Part print with two shaded views. Sizes in mm from the minimum x, y, z corner. A direction names the side the tool comes from. Round coordinates to 2 decimals unless told otherwise and drop trailing zeros. Write each loop counter-clockwise with the first axis right and the second up, starting at its lowest first coordinate (ties: lowest second). Pieces come first, ordered by that corner, then holes. Notation, with made-up numbers: (1.5, 15) - (45.5, 15) arc R17 ccw to (45.5, 20) - close; hole circle Ø3 at (-13, 48). An arc over 180 degrees is marked (long way). Answer as a JSON object with one key per item and string values. Group by question number.
Item 1: Flat gauge pins, fed straight in: pin 1 (1.7 mm diameter, centred on x = 13.25, y = 1.85, fed in from +Z); pin 2 (1.4 mm diameter, centred on x = 3.25, y = 1.85, fed in from +Z). Where does each tip first touch, or does it go through?
Item 2: Slice it at B-B, the plane y = 2.9. List the corners of the cut face in (x, z), then the cut area to 4 significant figures.
Item 3: Two-plate mould, pull along X, no slides. Class the marked faces 1, 2 and 3: +X half, -X half, draft (parallel to the pull), parting line (faces both ways), or undercut.
Item 4: Probe line 1 (X direction, y = 1.85, z = 5.3); line 2 (Y direction, x = 13.25, z = 2.5); line 3 (Z direction, x = 2.5, y = 0.8). List the from-to ranges inside material, lowest first. Write a range as from..to.
Item 5: Slice it at A-A, the plane z = 6. List the corners of the cut face in (x, y).
Item 6: Slice it at C-C, the plane y = 0.55. List the corners of the cut face in (x, z), then the cut area to 3 significant figures.
Item 7: Which spindle directions (+Z, -Z, +X, -X, +Y, -Y) get a long thin tool onto all of the face, cutting with end or side? Do the marked faces 4 and 5. Say none if no direction does.
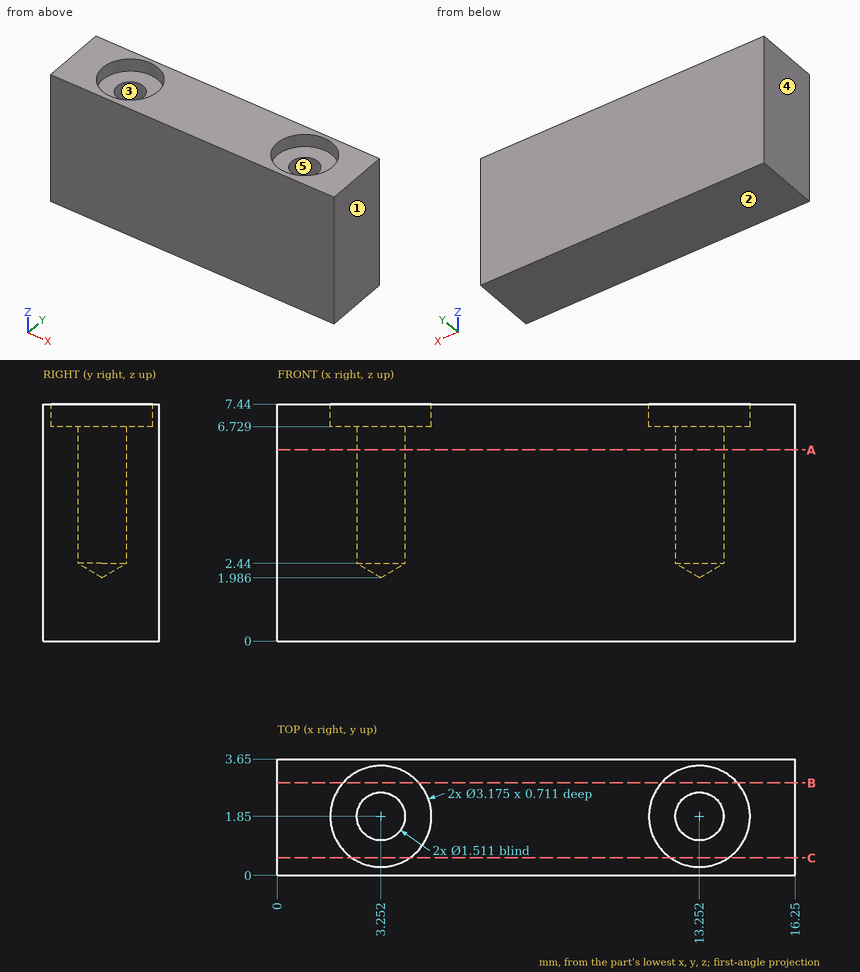
Geometry says:
{
 "1": {"pin 1": "stops at z = 6.73", "pin 2": "stops at z = 2.41"},
 "2": {"outline": "(0, 0) - (16.25, 0) - (16.25, 7.44) - (14.44, 7.44) - (14.44, 6.73) - (12.06, 6.73) - (12.06, 7.44) - (4.44, 7.44) - (4.44, 6.73) - (2.06, 6.73) - (2.06, 7.44) - (0, 7.44) - close", "area": "117.5 mm^2"},
 "3": {"face 1": "+X half", "face 2": "draft", "face 3": "undercut"},
 "4": {"line 1": "x = 0..2.5, 4.01..12.5, 14.01..16.25", "line 2": "y = 0..1.09, 2.61..3.65", "line 3": "z = 0..6.73"},
 "5": {"outline": "(0, 0) - (16.25, 0) - (16.25, 3.65) - (0, 3.65) - close; hole circle Ø1.51 at (3.25, 1.85); hole circle Ø1.51 at (13.25, 1.85)"},
 "6": {"outline": "(0, 0) - (16.25, 0) - (16.25, 7.44) - (14.16, 7.44) - (14.16, 6.73) - (12.34, 6.73) - (12.34, 7.44) - (4.16, 7.44) - (4.16, 6.73) - (2.34, 6.73) - (2.34, 7.44) - (0, 7.44) - close", "area": "118 mm^2"},
 "7": {"face 4": "+Z, -Z, -X, +Y, -Y", "face 5": "+Z"}
}
